The drawing under review shows one solid part. Ordinate dimensions are in mm from its lowest x, y, z. A direction names the side the tool comes from. Round coordinates to 2 decimals unless told otherwise and drop trailing zeros. Write each loop counter-clockwise with the first axis right and the second up, starting at its lowest first coordinate (ties: lowest second). Pieces come first, ordered by that corner, then holes. Notation, with made-up numbers: M 31.5,1 L 55.5,1 A8 cw 55.5,13 Z; hole C 85.25,77.5 d6. An arc over 180 degrees is marked long. Write item = value, one per line. Start each with the question number.
Item 1: To check wall thickness, follow line 1 along Y through (x, z) = (52.5, 91.5); line 2 along Z through (x, y) = (11, 685); line 3 along Z through (x, y) = (72, 269). State the ranges of each line that lie inside material, in increasing order.
Item 2: Take a section at D-D, the plane x = 32. Give the boundary of the cut face in (y, z).
Item 3: Take a section at A-A, the plane y = 629.5. Give the boundary of the cut face in (x, z), plus the area to 3 significant figures.
Item 4: Take a section at B-B, the plane x = 63.5. Give the boundary of the cut face in (y, z).
Item 5: Take a section at C-C, the plane z = 83.5. Give the boundary of the cut face in (x, y).
Item 6: For pin 1 Ø5 at (x, z) = (109.5, 14) entering from -Y; pin 2 Ø4 at (x, y) = (53.5, 279) entering from -Z, all flat-tipped, find the tip position at first contact; note any pin that passes through.
Item 7: Tool access review of the marked faces 1 and 2: name each direction out of +Z, -Z, +X, -X, +Y, -Y from which nothing blocks a thin tool from reaching the whole face with its end or side.
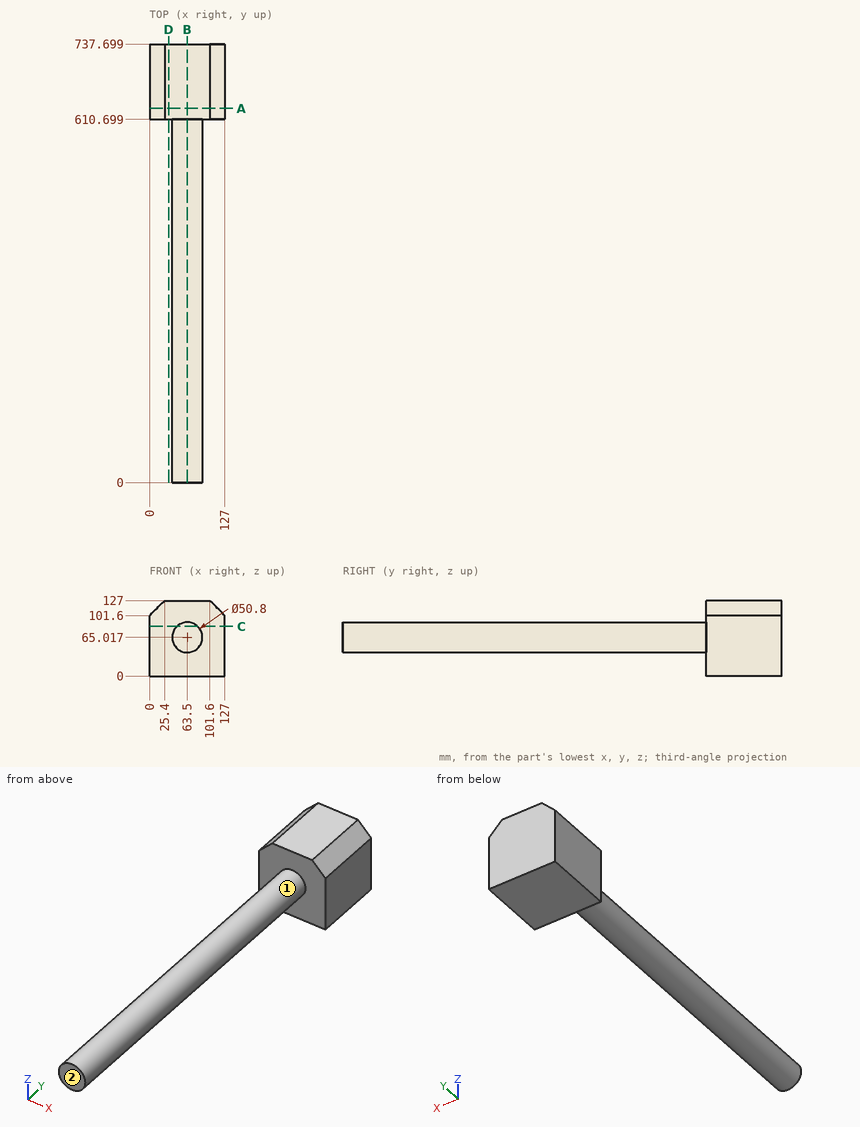
Response values:
q1.line_1 = 610.7 to 737.7
q1.line_2 = 0 to 112.6
q1.line_3 = 41.08 to 88.95
q2.outline = M 610.7,0 L 737.7,0 L 737.7,127 L 610.7,127 Z
q3.outline = M 0,0 L 127,0 L 127,101.6 L 101.6,127 L 25.4,127 L 0,101.6 Z
q3.area = 15,500 mm2
q4.outline = M 0,39.62 L 610.7,39.62 L 610.7,0 L 737.7,0 L 737.7,127 L 610.7,127 L 610.7,90.42 L 0,90.42 Z
q5.outline = M 0,610.7 L 46.08,610.7 L 46.08,0 L 80.92,0 L 80.92,610.7 L 127,610.7 L 127,737.7 L 0,737.7 Z
q6.pin_1 = 610.7
q6.pin_2 = 40.91
q7.face_1 = -Y
q7.face_2 = +Z, -Z, +X, -X, -Y
